Can you work these out from the model? Positions are in its coordinate system, mm. A direction names the side the tool comes from. Give positions to 0.01 mm unless a question says otherwise; leave off trailing zeros. Loops run counter-clockwise (first coordinate to the right, second up) from the corner with the lowest first, then second, coordinate; pieces in that order, holes last. Notation, with made-up numbers: (-35.5, 31.25) - (6.5, 31.25) arc R10 ccw to (6.5, 36.25) - close; hole circle Ø1 at (51, -5.5). An arc over 180 degrees is marked (long way). Answer as a JSON object with one key per item and string values.
```python
from build123d import *

# Parameters (mm, degrees)
SKETCH_1_W          = 107.889647592
SKETCH_1_H          = 93.399614016
EXTRUDE_1_DEPTH     = 2
SKETCH_2_R          = 11.639752959
EXTRUDE_2_DEPTH     = 30
SKETCH_3_R          = 10.388227947
CUT_EXTRUDE_1_DEPTH = 30


with BuildPart() as part:
    # 草图1 → 凸台-拉伸1 (new body)
    with BuildSketch(Plane(origin=(0, 0, 0), x_dir=(1, 0, 0), z_dir=(0, 1, 0))):
        with Locations((-9.950986914, -10.649301785)):
            Rectangle(SKETCH_1_W, SKETCH_1_H)
    extrude(amount=EXTRUDE_1_DEPTH)

    # 草图2 → 凸台-拉伸2 (add)
    with BuildSketch(Plane(origin=(0, 2, 0), x_dir=(1, 0, 0), z_dir=(0, 1, 0))):
        with Locations((-47.461132716, 22.11962872)):
            Circle(SKETCH_2_R)
    extrude(amount=EXTRUDE_2_DEPTH)

    # 草图3 → 切除-拉伸1 (cut)
    with BuildSketch(Plane(origin=(0, 2, 0), x_dir=(1, 0, 0), z_dir=(0, 1, 0))):
        with Locations((-9.699240969, -12.453481057)):
            Circle(SKETCH_3_R)
    extrude(amount=-CUT_EXTRUDE_1_DEPTH, mode=Mode.SUBTRACT)

    # 草图6 → 旋转4 (revolve)
    with BuildSketch(Plane(origin=(0, 0, 0), x_dir=(0, 0, -1), z_dir=(1, 0, 0))):
        with BuildLine():
            Line((-46.832059877, 2), (-42.473160934, 2))
            ThreePointArc((-42.473160934, 2), (-37.085265533, 13.236067977), (-46.832059877, 21))
            Line((-46.832059877, 21), (-46.832059877, 2))
        make_face()
    revolve(axis=Axis((0, 24.008191083, 46.832059877), (0, -1, 0)))

    # 草图7 → 旋转5 (revolve)
    with BuildSketch(Plane.XY):
        Polygon((16.639758733, 2), (29.897679802, 32.14170616), (29.897679802, 2), align=None)
    revolve(axis=Axis((29.897679802, 32.14170616, 0), (0, -1, 0)))


solid = part.part
```
1) Imagine slicing it at B-B on y = 24.5. Write out the boundary of the cut face in (x, z), and give its area (3 significant figures).
Check sheet entries:
{"outline": "circle Ø23.28 at (-47.46, -22.12); circle Ø6.72 at (29.9, 0)", "area": "461 mm2"}
2) Imagine slicing it at C-C on x = -30. Write out the boundary of the cut face in (y, z).
Check sheet entries:
{"outline": "(0, -36.05) - (2, -36.05) - (2, 57.35) - (0, 57.35) - close"}
3) Imagine slicing it at A-A on x = -7. Write out the boundary of the cut face in (y, z), and give its area (3 significant figures).
Check sheet entries:
{"outline": "(0, -36.05) - (2, -36.05) - (2, 2.42) - (0, 2.42) - close; (0, 22.48) - (2, 22.48) - (2, 57.35) - (0, 57.35) - close; circle Ø14.28 at (11, 46.83)", "area": "307 mm2"}
4) Imagine slicing it at D-D on z = 44.5. Write out the boundary of the cut face in (x, y), and give its area (3 significant figures).
Check sheet entries:
{"outline": "(-63.9, 0) - (43.99, 0) - (43.99, 2) - (3.68, 2) arc R9.72 ccw (long way) to (-3.68, 2) - (-63.9, 2) - close", "area": "509 mm2"}
5) If we mould it in two halves opening along Z, with no side actions, what happens to faces 3 (the flat face through (-11, 0, 0)), 4 (the cylindrical face through (0.2, 1, 9.3)), 5 (the conical face through (25.22, 20.63, 1.94))? For each: released by +Z, released by -Z, zero draft, split by the parting line, or undercut.
Check sheet entries:
{"face 3": "zero draft", "face 4": "undercut", "face 5": "split by the parting line"}
6) I need wall thicknesses on L1, parallel to Y at x = 31, z = 13.5; L2, parallel to Z at x = 22, y = 10.5; L3, parallel to Z at x = -53, y = 29.5. Which ranges of each line are inside material? Lowest first, please.
Check sheet entries:
{"L1": "0 to 2", "L2": "-5.31 to 5.31", "L3": "-32.36 to -11.88"}
7) Which directions (+Z, -Z, +X, -X, +Y, -Y) give clear straight access to the entire face, cutting with the end or side of a thin tool? Please do faces 1 (the cylindrical face through (-36.36, 16.79, -25.62)), 2 (the flat face through (-48, 32, -22)).
Check sheet entries:
{"face 1": "+Y", "face 2": "+Z, -Z, +X, -X, +Y"}
8) I'm going to push flat-ended pins straight in: P1, Ø2, axis at x = 29, y = 25, coming from the -Z side; P2, Ø18.5, axis at x = -49.5, z = -27, coming from the +Y side; P3, Ø12, axis at y = 9.5, z = -2.5, coming from the +X side. Where does each tip first touch, or does it pass through?
Check sheet entries:
{"P1": "z = -3.51", "P2": "y = 32", "P3": "x = 42.38"}
